```python
from build123d import *

# Parameters (mm, degrees)
SKETCH_1_W          = 3
SKETCH_1_H          = 46
SKETCH_1_W_2        = 4
SKETCH_1_H_2        = 4
EXTRUDE_1_DEPTH     = 100
SKETCH_2_W          = 8
SKETCH_2_H          = 8
CUT_EXTRUDE_1_DEPTH = 212.324395184


with BuildPart() as part:
    # Эскиз1 → Бобышка-Вытянуть1 (new, symmetric)
    with BuildSketch(Plane.XY):
        with Locations((1.5, 23)):
            Rectangle(SKETCH_1_W, SKETCH_1_H)
        with Locations((-2, 23)):
            Rectangle(SKETCH_1_W_2, SKETCH_1_H)
        Polygon((-4, 50), (0, 50), (3, 50), (17, 50), (17, 36), (20, 36), (20, 53), (0, 53), (-20, 53), (-20, 36), (-17, 36), (-17, 50), align=None)
        with Locations((-2, 48)):
            Rectangle(SKETCH_1_W_2, SKETCH_1_H_2)
        Polygon((-13, 46), (-4, 46), (-4, 50), (-17, 50), (-17, 36), (-13, 36), align=None)
        Polygon((3, 50), (3, 46), (13, 46), (13, 36), (17, 36), (17, 50), align=None)
        with Locations((1.5, 48)):
            Rectangle(SKETCH_1_W, SKETCH_1_H_2)
        Polygon((3, 0), (0, 0), (-4, 0), (-35, 0), (-35, 16), (-25, 16), (-25, 20), (-39, 20), (-39, -4), (35, -4), (35, 0), align=None)
        Polygon((35, -8), (35, -4), (-39, -4), (-39, 20), (-25, 20), (-25, 24), (-43, 24), (-43, -8), align=None)
    extrude(amount=EXTRUDE_1_DEPTH, both=True)

    # Эскиз2 → Вырез-Вытянуть1 (cut, through all)
    with BuildSketch(Plane.XY.offset(100)):
        with Locations((31, -4)):
            Rectangle(SKETCH_2_W, SKETCH_2_H)
    extrude(amount=-CUT_EXTRUDE_1_DEPTH, mode=Mode.SUBTRACT)


solid = part.part
```
Check sheet for the modelled part. Datum: model origin and axes. Units: mm. A direction names the side the tool comes from. Round coordinates to 2 decimals unless told otherwise and drop trailing zeros. Order: outer loops, then holes, each group sorted by start corner. A loop starts at its lowest first (then second) coordinate and runs counter-clockwise, first axis right, second up. Notation, with made-up numbers: (74.5, -7) -> (82.5, -7) arc R14 ccw to (82.5, 13) -> close; hole circle Ø2 at (61.5, -26). An arc over 180 degrees is marked (long way). One line per item, written item: value. Start each with the question number.
Q1. Gauge pin test, flat ends, axial feed: pin 1 Ø5 at (y, z) = (42.5, -46) entering from -X; pin 2 Ø1 at (y, z) = (46, -28) entering from +X; pin 3 Ø5 at (x, z) = (-27, -44) entering from +Y. Record the tip position at first contact, or that the pin passes through.
Q2. Cross-section at C-C (y = 28.5). Record the boundary of the cut face in (x, z), and give its area (3 significant figures).
Q3. Cross-section at B-B (z = 72.5). Record the boundary of the cut face in (x, y), and give its area (3 significant figures).
Q4. Mould release check, pull along X, two halves, no side actions. Record for faces 5 (the face through (15, 0, 1)), 6 (the face through (-43, 8, 1)), 7 (the face through (3, 23, 1)): pulls with the +X half, pulls with the -X half, needs draft (parallel to the pull), parting line crosses it, or undercut.
Q5. Cross-section at A-A (x = -27). Record the boundary of the cut face in (y, z), and give its area (3 significant figures).
Q6. Set-up check for faces 1 (the face through (-17, 36, 1)), 2 (the face through (-20, 45, 1)), 3 (the face through (-25, 20, 1)), 4 (the face through (8, 46, 1)): record each of +Z, -Z, +X, -X, +Y, -Y from which the full face is reachable in a straight line by a thin tool's end or side.
Q7. Thickness scan on line 1 (X direction, y = 40, z = 28); line 2 (Y direction, x = -12, z = 45); line 3 (Y direction, x = -29.5, z = -65.5). Record the ranges inside material, lowest first.
Q8. Cross-section at D-D (x = -17). Record the boundary of the cut face in (y, z), and give its area (3 significant figures).
Completed:
1. pin 1: stops at x = -20
1. pin 2: stops at x = 20
1. pin 3: stops at y = 24
2. outline: (-4, -100) -> (3, -100) -> (3, 100) -> (-4, 100) -> close
2. area: 1,400 mm²
3. outline: (-43, -8) -> (27, -8) -> (27, 0) -> (3, 0) -> (3, 46) -> (13, 46) -> (13, 36) -> (20, 36) -> (20, 53) -> (-20, 53) -> (-20, 36) -> (-13, 36) -> (-13, 46) -> (-4, 46) -> (-4, 0) -> (-35, 0) -> (-35, 16) -> (-25, 16) -> (-25, 24) -> (-43, 24) -> close
3. area: 1,570 mm²
4. face 5: needs draft
4. face 6: pulls with the -X half
4. face 7: undercut
5. outline: (-8, -100) -> (0, -100) -> (0, 100) -> (-8, 100) -> close; (16, -100) -> (24, -100) -> (24, 100) -> (16, 100) -> close
5. area: 3,200 mm²
6. face 1: +Z, -Z, -X
6. face 2: +Z, -Z, -X, +Y
6. face 3: +Z, -Z, +Y
6. face 4: +Z, -Z
7. line 1: x = -20 to -13, -4 to 3, 13 to 20
7. line 2: y = -8 to 0, 46 to 53
7. line 3: y = -8 to 0, 16 to 24
8. outline: (-8, -100) -> (0, -100) -> (0, 100) -> (-8, 100) -> close; (36, -100) -> (53, -100) -> (53, 100) -> (36, 100) -> close
8. area: 5,000 mm²
